The listing builds one solid part. Answer for the finished solid, in the listing's coordinates (mm). A direction names the side the tool comes from. Give positions to 0.01 mm unless a question says otherwise; leave off trailing zeros. Loops run counter-clockwise (first coordinate to the right, second up) from the corner with the lowest first, then second, coordinate; pieces in that order, holes last. Notation, with made-up numbers: M 49.5,88 L 58.5,88 A15 cw 58.5,94 Z; hole C 29.25,21.25 d2. An arc over 180 degrees is marked long. One line per item, written item: value. Start each with the question number.
Q1. A cutting plane is placed at D-D, the plane y = -5. Determine the outline of the cut face in (x, z), and give its area (3 significant figures).
Q2. A cutting plane is placed at C-C, the plane z = 18. Determine the outline of the cut face in (x, y).
Q3. For faces 1 (the flat face through (-22.3, -12.52, 22.96)), 2 (the flat face through (-41.436, -30, 21)), 3 (the flat face through (-50.773, -30, 21)), determine the directions among +Z, -Z, +X, -X, +Y, -Y from which every point of the face is accessible in a straight line to the end or side of a thin tool.
Q4. A cutting plane is placed at B-B, the plane x = -47.5. Determine the outline of the cut face in (y, z), and give its area (3 significant figures).
Q5. Flat-ended cylindrical pins translate along their axes: pin 1 (5 mm diameter, centred on x = -36.5, z = 19, fed in from -Y); pin 2 (6.5 mm diameter, centred on x = -59.5, y = -30, fed in from +Z); pin 3 (12 mm diameter, centred on y = -17, z = 27, fed in from +X). Find the tip coordinate at first contact, or state that the pin passes through.
Q6. Consider L1, parallel to X at y = -27, z = 27.25; L2, parallel to Z at x = -51, y = -30.5; L3, parallel to Y at x = -35, z = 21.25. Determine where each line is inside the solid, lowest interval first.
Q7. A cutting plane is placed at A-A, the plane y = -35. Determine the outline of the cut face in (x, z), and give its area (3 significant figures).
from build123d import *

# Parameters (mm, degrees)
F1_DEPTH = 25.4
F2_W     = 50.8
F2_H     = 12.7
F3_DEPTH = 12.7
F4_W     = 9.3365699251
F4_H     = 14.1990316571
F5_DEPTH = 12.7
F7_DEPTH = 25.4


# Not quite as in the source:
# - a feature names something its author has since deleted; it is built from what else it names


with BuildPart() as f1:
    # F0 (on Front) → F1 (new body)
    with BuildSketch(Plane.XZ):
        Polygon((-66.8362646442, 30.1552314789), (-66.8362646442, 3.2561998218), (-16.0362646442, 3.2561998218), (-16.0362646442, 15.9561998218), (-28.7362646442, 30.1552314789), align=None)
    extrude(amount=F1_DEPTH)

    # F2 (on face) → F3 (join)
    with BuildSketch(Plane.XZ.offset(25.4)):
        with Locations((-41.4362646442, 9.6061998218)):
            Rectangle(F2_W, F2_H)
    extrude(amount=F3_DEPTH)

    # F4 (on face) → F5 (join)
    with BuildSketch(Plane.XZ.offset(25.4)):
        with Locations((-46.1045496067, 23.0557156503)):
            Rectangle(F4_W, F4_H)
    extrude(amount=F5_DEPTH)

    # F6 (on face) → F7 (cut)
    with BuildSketch(Plane.YZ.offset(-41.4362646442)):
        Polygon((-38.1, 15.9561998218), (-25.4, 30.1552314789), (-38.1, 30.1552314789), align=None)
    extrude(amount=-F7_DEPTH, mode=Mode.SUBTRACT)


solid = f1.part
Answer block:
1. outline: M -66.84,3.26 L -16.04,3.26 L -16.04,15.96 L -28.74,30.16 L -66.84,30.16 Z
1. area: 1,280 mm^2
2. outline: M -66.84,-25.4 L -50.77,-25.4 L -50.77,-36.27 L -41.44,-36.27 L -41.44,-25.4 L -17.86,-25.4 L -17.86,0 L -66.84,0 Z
3. face 1: +Z, +X, +Y, -Y
3. face 2: +Z, +X, -Y
3. face 3: +Z, -X, -Y
4. outline: M -38.1,3.26 L 0,3.26 L 0,30.16 L -25.4,30.16 L -38.1,15.96 Z
4. area: 935 mm^2
5. pin 1: y = -25.4
5. pin 2: z = 15.96
5. pin 3: x = -20.55
6. L1: -50.77 to -41.44
6. L2: 3.26 to 15.96
6. L3: -25.4 to 0
7. outline: M -66.84,3.26 L -16.04,3.26 L -16.04,15.96 L -41.44,15.96 L -41.44,19.42 L -50.77,19.42 L -50.77,15.96 L -66.84,15.96 Z
7. area: 678 mm^2
